For this review, use the dimensioned drawing (mm, ordinates from the lowest corner) and the shaded views. Coordinates: 2 decimals unless noted, no trailing zeros. Write each loop counter-clockwise with the first axis right and the second up, starting at its lowest first coordinate (ties: lowest second). Pieces come first, ordered by that corner, then holes. Notation, with made-up numbers: M 25.5,89.5 L 34.5,89.5 A31 cw 34.5,118.5 Z; hole C 6,16 d1. An arc over 180 degrees is marked long. One line per question, with ' | ' between items.
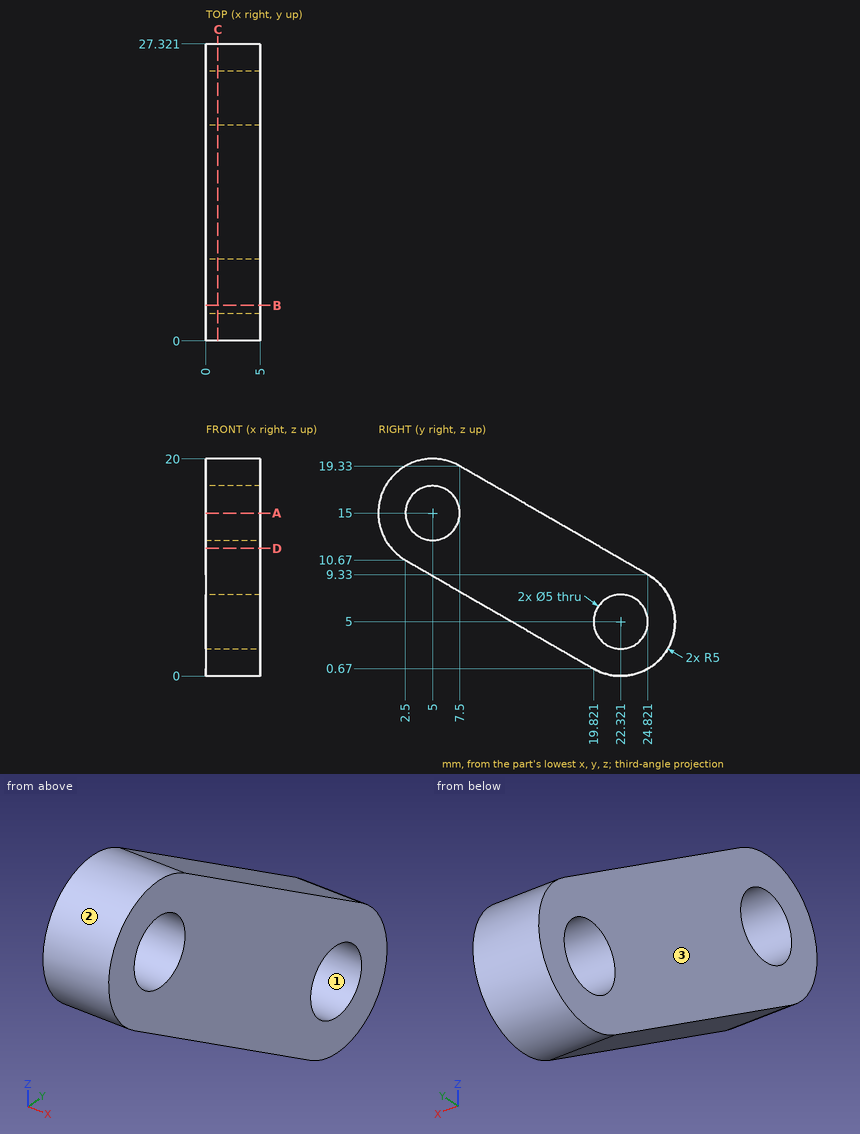
1. Draft analysis for pull direction Z (two halves, no side actions). For the marked faces 1, 2 and 3, state which applies: pulls with the +Z half, pulls with the -Z half, needs draft (parallel to the pull), parting line crosses it, or undercut.
Answer sheet:
face 1: undercut | face 2: parting line crosses it | face 3: needs draft
2. Take a section at A-A (z = 15). Write out the cut boundary in (x, y).
Answer sheet:
outline: M 0,0 L 5,0 L 5,2.5 L 0,2.5 Z; M 0,7.5 L 5,7.5 L 5,15 L 0,15 Z
3. To check wall thickness, follow line 1 along Z through (x, y) = (2.95, 24.5) (1 decimal); line 2 along Z through (x, y) = (3, 22.75) (1 decimal); line 3 along Y through (x, z) = (0.55, 17.25) (1 decimal). State the ranges of each line that lie inside material, in increasing order. Write a range as [from, to].
Answer sheet:
line 1: [0.5, 3.8], [6.2, 9.5] | line 2: [0, 2.5], [7.5, 10.5] | line 3: [0.5, 3.9], [6.1, 11.1]
4. Take a section at D-D (z = 11.75). Write out the cut boundary in (x, y).
Answer sheet:
outline: M 0,1.2 L 5,1.2 L 5,20.63 L 0,20.63 Z
5. Insertion check: pin 1 Ø1 at (x, y) = (3.5, 16) entering from +Z; pin 2 Ø1 at (x, z) = (1.5, 17) entering from +Y (1 decimal); pin 3 Ø3 at (x, y) = (1.5, 4.5) entering from -Z. Each pin has a flat end and moves straight along its axis. Give the tip position at first contact, or say it passes through.
Answer sheet:
pin 1: z = 14.71 | pin 2: y = 12.4 | pin 3: z = 8.65
6. Take a section at C-C (x = 1.1). Write out the cut boundary in (y, z).
Answer sheet:
outline: M 2.5,10.67 L 19.82,0.67 A5 ccw 24.82,9.33 L 7.5,19.33 A5 ccw Z; hole C 5,15 d5; hole C 22.32,5 d5
7. Take a section at B-B (y = 3.25). Write out the cut boundary in (x, z) (1 decimal).
Answer sheet:
outline: M 0,10.2 L 5,10.2 L 5,13.2 L 0,13.2 Z; M 0,16.8 L 5,16.8 L 5,19.7 L 0,19.7 Z
